The drawing under review shows one solid part. Ordinate dimensions are in mm from its lowest x, y, z. A direction names the side the tool comes from. Round coordinates to 2 decimals unless told otherwise and drop trailing zeros. Order: outer loops, then holes, each group sorted by start corner. A loop starts at its lowest first (then second) coordinate and runs counter-clockwise, first axis right, second up. Notation, with made-up numbers: M 26,15.5 L 46,15.5 A26 ccw 46,31.5 Z; hole C 64,86 d8. An arc over 180 degrees is marked long. Use a Markdown table: item, result.
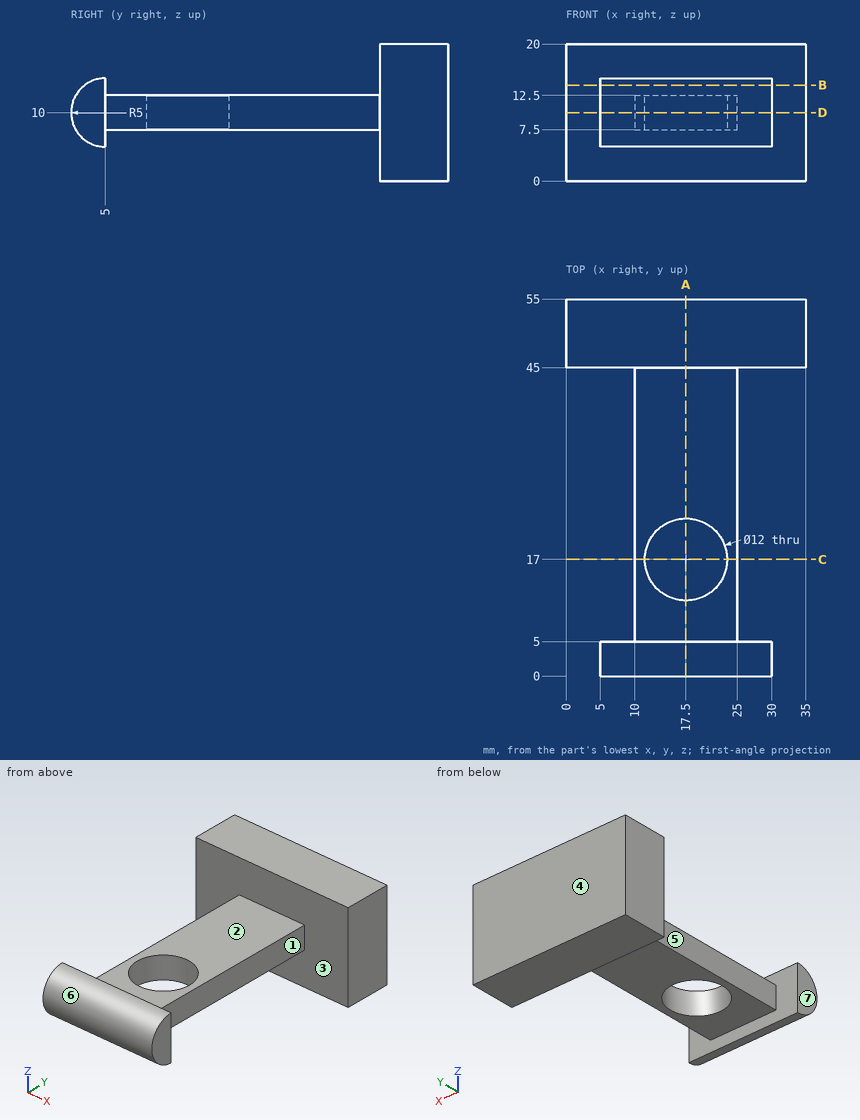
Q1. Draft analysis for pull direction Y (two halves, no side actions). For the marked faces 4, 5, 6 and 7, state which applies: pulls with the +Y half, pulls with the -Y half, needs draft (parallel to the pull), parting line crosses it, or undercut.
Determined:
| item | result |
|---|---|
| face 4 | pulls with the +Y half |
| face 5 | undercut |
| face 6 | pulls with the -Y half |
| face 7 | needs draft |
Q2. Add section B-B (z = 14). Write out the cut boundary in (x, y).
Determined:
| item | result |
|---|---|
| outline | M 0,45 L 35,45 L 35,55 L 0,55 Z; M 5,2 L 30,2 L 30,5 L 5,5 Z |
Q3. Wall thickness on line 1 along Y through (x, z) = (17.5, 10.35); line 2 along Z through (x, y) = (21, 22.5); line 3 along Y through (x, z) = (11, 15.5): over which ranges is each line inside the solid? List them lowest first. Write a range as [from, to].
Determined:
| item | result |
|---|---|
| line 1 | y = [0.01, 11], [23, 55] |
| line 2 | z = [7.5, 12.5] |
| line 3 | y = [45, 55] |
Q4. Clearance check with flat-ended pins moving along their axes: pin 1 (4 mm diameter, centred on y = 17, z = 9, fed in from -X); pin 2 (1.5 mm diameter, centred on y = 1.5, z = 11, fed in from +X); pin 3 (12 mm diameter, centred on x = 21, y = 16.5, fed in from +Z); pin 4 (11 mm diameter, centred on x = 17.5, y = 17, fed in from +Z). State where each tip first meets the part, or that it passes through.
Determined:
| item | result |
|---|---|
| pin 1 | stops at x = 10 |
| pin 2 | stops at x = 30 |
| pin 3 | stops at z = 12.5 |
| pin 4 | passes through |
Q5. Add section A-A (x = 17.5). Write out the cut boundary in (y, z), then the cut area to 3 significant figures.
Determined:
| item | result |
|---|---|
| outline | M 5,5 L 5,7.5 L 11,7.5 L 11,12.5 L 5,12.5 L 5,15 A5 ccw Z; M 23,7.5 L 45,7.5 L 45,0 L 55,0 L 55,20 L 45,20 L 45,12.5 L 23,12.5 Z |
| area | 379 mm^2 |
Q6. Add section C-C (y = 17). Write out the cut boundary in (x, z), then the cut area to 3 significant figures.
Determined:
| item | result |
|---|---|
| outline | M 10,7.5 L 11.5,7.5 L 11.5,12.5 L 10,12.5 Z; M 23.5,7.5 L 25,7.5 L 25,12.5 L 23.5,12.5 Z |
| area | 15.0 mm^2 |
Q7. Machinability: for the marked faces 1, 2 and 3, which of the approach directions +Z, -Z, +X, -X, +Y, -Y give a long, thin tool a straight path to every point of the face, cutting with its end or side? Answer none if there is none.
Determined:
| item | result |
|---|---|
| face 1 | +Z, -Z, +X |
| face 2 | +Z, +X, -X |
| face 3 | none |
Q8. Add section D-D (z = 10). Write out the cut boundary in (x, y), then the cut area to 3 significant figures.
Determined:
| item | result |
|---|---|
| outline | M 0,45 L 10,45 L 10,5 L 5,5 L 5,0 L 30,0 L 30,5 L 25,5 L 25,45 L 35,45 L 35,55 L 0,55 Z; hole C 17.5,17 d12 |
| area | 962 mm^2 |
